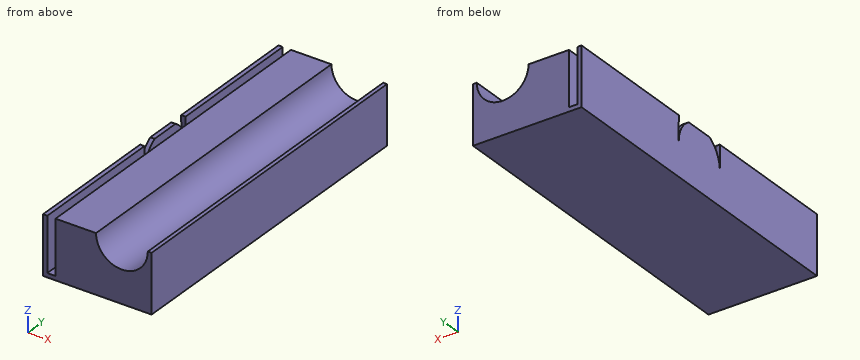
Autodesk Fusion 360 part; units mm, degrees
sketch "Sketch1" plane through (0, 0, 0) normal (0, 0, 1) x (1, 0, 0)
  line L0 (0, 0) -> (13, 0)
  line L1 (13, 0) -> (13, 40)
  line L2 (13, 40) -> (0, 40)
  line L3 (0, 40) -> (0, 0)
  dimension "d1" = 13
  dimension "d2" = 40
extrude "Extrude1" add sketch "Sketch1" along normal blind 7 and the other way blind 0
sketch "Sketch2" plane through (0, 0, 0) normal (0, -1, 0) x (1, 0, 0)
  line L0 (0, 0) -> (13, 0)
  line L1 (13, 0) -> (13, 7)
  line L2 (13, 7) -> (0, 7)
  line L3 (0, 7) -> (0, 0)
  circle A0 centre (9.4477, 7.0008) radius 3.1
  dimension "d5" = 6.2
extrude "Extrude2" cut sketch "Sketch2" against normal blind 41 contours L2 A0 picked at (8.7012, 5.7442)
sketch "Sketch4" plane through (0, 0, 7) normal (0, 0, 1) x (-1, 0, 0)
  line L0 (-6.3477, 0) -> (-6.3477, -40)
  line L1 (-6.3477, -40) -> (0, -40)
  line L2 (0, -40) -> (0, 0)
  line L3 (0, 0) -> (-6.3477, 0)
  line L4 (-0.517, -40) -> (-1.5, -40)
  line L5 (-1.5, -40) -> (-1.5, 0)
  line L6 (-1.5, 0) -> (-0.517, 0)
  line L7 (-0.517, 0) -> (-0.517, -40)
extrude "Extrude4" cut sketch "Sketch4" against normal blind 6.5 contours L1 L3 L4 L5 L6 L7
sketch "Sketch5" plane through (0, 0, 0) normal (-1, 0, 0) x (0, -1, 0)
  line L0 (-40, 0) -> (0, 0)
  line L1 (0, 0) -> (0, 7)
  line L2 (0, 7) -> (-40, 7)
  line L3 (-40, 7) -> (-40, 0)
  circle A0 centre (-20, 3.9772) radius 3.5
  line L4 (-23.5, 3.9917) -> (-23.4875, 7)
  line L5 (-16.5, 3.9917) -> (-16.5125, 7)
  dimension "d15" = 7
extrude "Extrude5" cut sketch "Sketch5" against normal blind 1 contours L2 A0 L4 | L2 A0 L5 | L2 A0 picked at (-19.7165, 7.2777)
Design review of the part built by this model. Coordinates are the model's own, in mm. Round coordinates to 2 decimals unless told otherwise and drop trailing zeros. Write each loop counter-clockwise with the first axis right and the second up, starting at its lowest first coordinate (ties: lowest second). Pieces come first, ordered by that corner, then holes. Notation, with made-up numbers: (33.5, 55.25) -> (50.5, 55.25) arc R20 cw to (50.5, 80.25) -> close; hole circle Ø4 at (0, 36). An arc over 180 degrees is marked (long way). Answer in a Markdown table with one row per item.
Q1. Take a section at A-A, the plane z = 3.5. State the section outline as (x, y) points.
The answers:
| item | result |
|---|---|
| outline | (0, 0) -> (0.52, 0) -> (0.52, 40) -> (0, 40) -> close; (1.5, 0) -> (13, 0) -> (13, 40) -> (1.5, 40) -> close |
Q2. Clearance check with a flat-ended pin moving along its axis: pin 1 Ø0.8 at (x, y) = (1, 28) entering from +Z. State where the tip first meets the part, or that it passes through.
The answers:
| item | result |
|---|---|
| pin 1 | z = 0.5 |
Q3. Take a section at D-D, the plane x = 11. State the section outline as (y, z) points.
The answers:
| item | result |
|---|---|
| outline | (0, 0) -> (40, 0) -> (40, 4.32) -> (0, 4.32) -> close |
Q4. Take a section at B-B, the plane y = 12.5. State the section outline as (x, z) points.
The answers:
| item | result |
|---|---|
| outline | (0, 0) -> (13, 0) -> (13, 7) -> (12.55, 7) arc R3.1 cw to (6.35, 7) -> (1.5, 7) -> (1.5, 0.5) -> (0.52, 0.5) -> (0.52, 7) -> (0, 7) -> close |
Q5. To check wall thickness, follow L1, parallel to X at y = 29, z = 5.25; L2, parallel to X at y = 2.5, z = 2.75; L3, parallel to X at y = 27.5, z = 5. State the ranges of each line that lie inside material, in increasing order. Write a range as [from, to].
The answers:
| item | result |
|---|---|
| L1 | [0, 0.52], [1.5, 6.89], [12.01, 13] |
| L2 | [0, 0.52], [1.5, 13] |
| L3 | [0, 0.52], [1.5, 7.08], [11.82, 13] |
Q6. Take a section at C-C, the plane z = 6.25. State the section outline as (x, y) points, then the cut area to 3 significant figures.
The answers:
| item | result |
|---|---|
| outline | (0, 0) -> (0.52, 0) -> (0.52, 16.51) -> (0, 16.51) -> close; (0, 17.34) -> (0.52, 17.34) -> (0.52, 22.66) -> (0, 22.66) -> close; (0, 23.49) -> (0.52, 23.49) -> (0.52, 40) -> (0, 40) -> close; (1.5, 0) -> (6.44, 0) -> (6.44, 40) -> (1.5, 40) -> close; (12.46, 0) -> (13, 0) -> (13, 40) -> (12.46, 40) -> close |
| area | 239 mm² |
